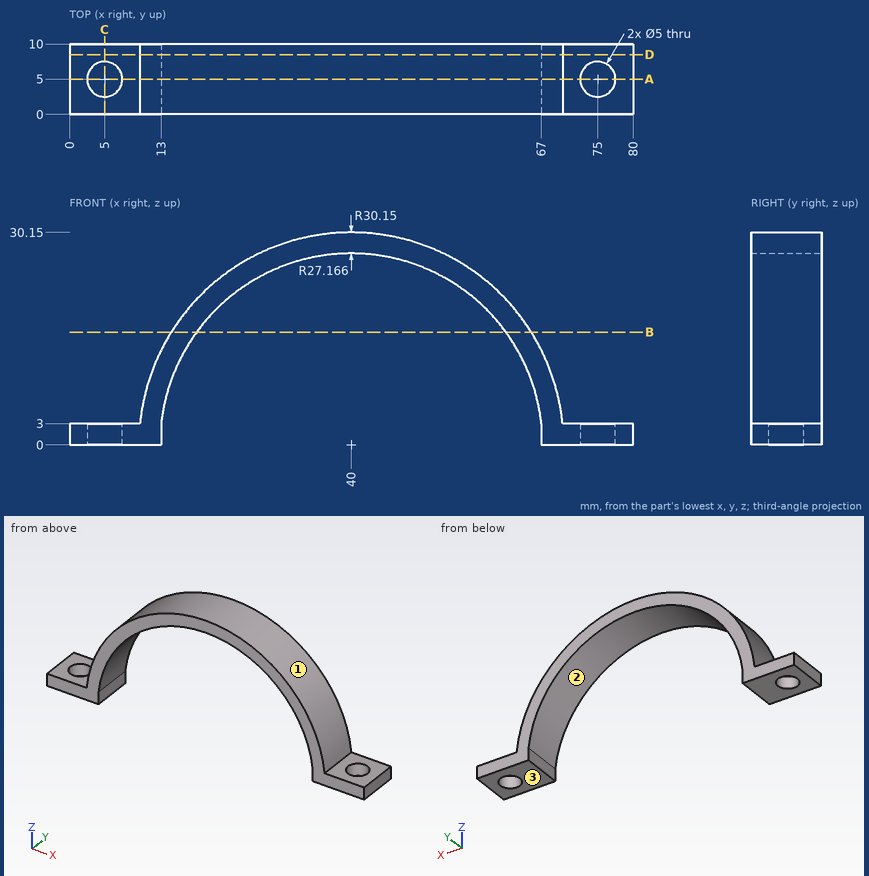
The drawing under review shows one solid part. Ordinate dimensions are in mm from its lowest x, y, z. Give positions to 0.01 mm unless a question says otherwise; leave off trailing zeros. Write each loop counter-clockwise with the first axis right and the second up, starting at its lowest first coordinate (ties: lowest second). Pieces come first, ordered by that corner, then holes. Notation, with made-up numbers: (62.5, 9.25) - (103.5, 9.25) arc R31 cw to (103.5, 46.25) - close; hole circle Ø1 at (11.25, 88.5). An arc over 180 degrees is marked (long way). Answer in a Markdown table with one row per item. Add a question column.
1. Draft analysis for pull direction X (two halves, no side actions). For the marked faces 1, 2 and 3, state which applies: +X half, -X half, draft (parallel to the pull), parting line (faces both ways), or undercut.
2. Wall thickness on line 1 along X through (y, z) = (5, 1.3); line 2 along Y through (x, z) = (5, 2); line 3 along X through (y, z) = (2.75, 3.5) (1 decimal): over which ranges is each line inside the solid? List them lowest first. Write a range as [from, to].
3. We need section D-D on y = 8.5. Write out the cut boundary in (x, z), then the cut area to 3 significant figures.
4. We need section A-A on y = 5. Write out the cut boundary in (x, z).
5. Insertion check: P1, Ø5, axis at x = 77, y = 5, coming from the +Z side; P2, Ø5, axis at y = 3.5, z = 21, coming from the -X side; P3, Ø3, axis at y = 2, z = 16.5, coming from the +X side; P4, Ø4.5, axis at x = 5, y = 5, coming from the +Z side. Each pin has a flat end and moves straight along its axis. Give the tip position at first contact, or say it passes through.
6. We need section C-C on x = 5. Write out the cut boundary in (y, z).
7. We need section B-B on z = 16. Write out the cut boundary in (x, y) (1 decimal).
Ans:
| question | item | result |
|---|---|---|
| 1 | face 1 | parting line |
| 1 | face 2 | undercut |
| 1 | face 3 | draft |
| 2 | line 1 | x = [0, 2.5], [7.5, 13], [67, 72.5], [77.5, 80] |
| 2 | line 2 | y = [0, 2.5], [7.5, 10] |
| 2 | line 3 | x = [10.1, 13.1], [66.9, 69.9] |
| 3 | outline | (0, 0) - (13, 0) - (13, 3) arc R27.17 cw to (67, 3) - (67, 0) - (80, 0) - (80, 3) - (70, 3) arc R30.15 ccw to (10, 3) - (0, 3) - close |
| 3 | area | 329 mm^2 |
| 4 | outline | (0, 0) - (2.5, 0) - (2.5, 3) - (0, 3) - close; (7.5, 0) - (13, 0) - (13, 3) arc R27.17 cw to (67, 3) - (67, 0) - (72.5, 0) - (72.5, 3) - (70, 3) arc R30.15 ccw to (10, 3) - (7.5, 3) - close; (77.5, 0) - (80, 0) - (80, 3) - (77.5, 3) - close |
| 5 | P1 | stops at z = 3 |
| 5 | P2 | stops at x = 16.19 |
| 5 | P3 | stops at x = 66.15 |
| 5 | P4 | passes through |
| 6 | outline | (0, 0) - (2.5, 0) - (2.5, 3) - (0, 3) - close; (7.5, 0) - (10, 0) - (10, 3) - (7.5, 3) - close |
| 7 | outline | (14.4, 0) - (18, 0) - (18, 10) - (14.4, 10) - close; (62, 0) - (65.6, 0) - (65.6, 10) - (62, 10) - close |
